```python
from build123d import *

# Parameters (mm, degrees)
BOSS_EXTRUDE1_DEPTH = 550
SKETCH2_W           = 99.516911358
SKETCH2_H           = 250
CUT_EXTRUDE1_DEPTH  = 596.064959308
SKETCH4_R           = 5
CUT_EXTRUDE2_DEPTH  = 20
SKETCH4_3_R         = 5
BOSS_EXTRUDE3_DEPTH = 2.5
BOSS_EXTRUDE4_START = 17.5
SKETCH4_5_R         = 5
BOSS_EXTRUDE4_DEPTH = 2.5
SKETCH4_7_R         = 1.240896304
BOSS_EXTRUDE5_DEPTH = 17.5
BOSS_EXTRUDE6_START = -150
SKETCH5_R           = 5
SKETCH5_R_2         = 1.5
BOSS_EXTRUDE6_DEPTH = 19.5
CUT_EXTRUDE5_START  = -167.5
SKETCH5_4_R         = 5
CUT_EXTRUDE5_DEPTH  = 2.5
CUT_EXTRUDE6_START  = -150
SKETCH5_6_R         = 5
CUT_EXTRUDE6_DEPTH  = 2.5
BOSS_EXTRUDE7_DEPTH = 2


with BuildPart() as part:
    # Sketch1 → Boss-Extrude1 (new body)
    with BuildSketch(Plane.XY):
        Polygon((0, 0), (-63.508529611, 110), (-61.222529611, 110), (0.966177285, 2.286), (200, 2.286), (200, 0), align=None)
    extrude(amount=BOSS_EXTRUDE1_DEPTH)

    # Sketch2 → Cut-Extrude1 (cut, through all)
    with BuildSketch(Plane(origin=(0, 2.286, 0), x_dir=(1, 0, 0), z_dir=(0, 1, 0))):
        with Locations((150.241544321, -275)):
            Rectangle(SKETCH2_W, SKETCH2_H)
    extrude(amount=-CUT_EXTRUDE1_DEPTH, mode=Mode.SUBTRACT)

    # Sketch4 → Cut-Extrude2 (cut)
    with BuildSketch(Plane.XY.offset(150)):
        with Locations((0.483088642, 1.143)):
            Circle(SKETCH4_R)
    cut_extrude2 = extrude(amount=CUT_EXTRUDE2_DEPTH, mode=Mode.SUBTRACT)

    # Sketch4_3 → Boss-Extrude3 (add)
    with BuildSketch(Plane.XY.offset(150)):
        with Locations((0.483088642, 1.143)):
            Circle(SKETCH4_3_R)
    boss_extrude3 = extrude(amount=BOSS_EXTRUDE3_DEPTH)

    # Sketch4_5 → Boss-Extrude4 (add)
    with BuildSketch(Plane.XY.offset(150).offset(BOSS_EXTRUDE4_START)):
        with Locations((0.483088642, 1.143)):
            Circle(SKETCH4_5_R)
    boss_extrude4 = extrude(amount=BOSS_EXTRUDE4_DEPTH)

    # Sketch4_7 → Boss-Extrude5 (add)
    with BuildSketch(Plane.XY.offset(150)):
        with Locations((0.483088642, 1.143)):
            Circle(SKETCH4_7_R)
    boss_extrude5 = extrude(amount=BOSS_EXTRUDE5_DEPTH)

    # Mirror1: Cut-Extrude2, Boss-Extrude3, Boss-Extrude4, Boss-Extrude5 across plane
    add(cut_extrude2.mirror(Plane.XY.offset(275)), mode=Mode.SUBTRACT)
    add(boss_extrude3.mirror(Plane.XY.offset(275)))
    add(boss_extrude4.mirror(Plane.XY.offset(275)))
    add(boss_extrude5.mirror(Plane.XY.offset(275)))

    # Sketch5 → Boss-Extrude6 (add)
    with BuildSketch(Plane.XY.offset(550).offset(BOSS_EXTRUDE6_START)):
        with Locations((-65.55265663, 107.5)):
            Circle(SKETCH5_R)
        with Locations((-65.55265663, 107.5)):
            Circle(SKETCH5_R_2, mode=Mode.SUBTRACT)
    boss_extrude6 = extrude(amount=-BOSS_EXTRUDE6_DEPTH)

    # Sketch5_4 → Cut-Extrude5 (cut)
    with BuildSketch(Plane.XY.offset(550).offset(CUT_EXTRUDE5_START)):
        with Locations((-65.55265663, 107.5)):
            Circle(SKETCH5_4_R)
    cut_extrude5 = extrude(amount=-CUT_EXTRUDE5_DEPTH, mode=Mode.SUBTRACT)

    # Sketch5_6 → Cut-Extrude6 (cut)
    with BuildSketch(Plane.XY.offset(550).offset(CUT_EXTRUDE6_START)):
        with Locations((-65.55265663, 107.5)):
            Circle(SKETCH5_6_R)
    cut_extrude6 = extrude(amount=-CUT_EXTRUDE6_DEPTH, mode=Mode.SUBTRACT)

    # Mirror2: Boss-Extrude6, Cut-Extrude5, Cut-Extrude6 across plane
    add(boss_extrude6.mirror(Plane.XY.offset(275)))
    add(cut_extrude5.mirror(Plane.XY.offset(275)), mode=Mode.SUBTRACT)
    add(cut_extrude6.mirror(Plane.XY.offset(275)), mode=Mode.SUBTRACT)

    # Sketch7 → Boss-Extrude7 (add)
    with BuildSketch(Plane.XY.offset(550)):
        with BuildLine():
            Line((32.714, 2.286), (35, 2.286))
            Line((35, 2.286), (35, 20))
            Line((35, 20), (15, 20))
            Line((15, 20), (19.696699141, 15.303300859))
            ThreePointArc((19.696699141, 15.303300859), (27.870125743, 16.929096494), (32.5, 10))
            ThreePointArc((32.5, 10), (31.929096494, 7.129874257), (30.303300859, 4.696699141))
            Line((30.303300859, 4.696699141), (32.714, 2.286))
        make_face()
        with BuildLine():
            Line((15, 20), (15, 2.286))
            Line((15, 2.286), (32.714, 2.286))
            Line((32.714, 2.286), (30.303300859, 4.696699141))
            ThreePointArc((30.303300859, 4.696699141), (19.696699141, 4.696699141), (19.696699141, 15.303300859))
            Line((19.696699141, 15.303300859), (15, 20))
        make_face()
        Polygon((15, 2.286), (15, 0), (35, 0), (32.714, 2.286), align=None)
        Polygon((32.714, 2.286), (35, 0), (35, 2.286), align=None)
    extrude(amount=BOSS_EXTRUDE7_DEPTH)


solid = part.part
```
Design review of the part built by this model. Coordinates are the model's own, in mm. A direction names the side the tool comes from. Coordinates: 2 decimals unless noted, no trailing zeros. Order: outer loops, then holes, each group sorted by start corner. A loop starts at its lowest first (then second) coordinate and runs counter-clockwise, first axis right, second up.
1) Mouldability with a two-part tool opening along Z and no side actions: class faces 3 (the flat face through (-33, 59, 550)), 4 (the flat face through (20, 17, 550)), 5 (the flat face through (2, 0, 382.5)) as +Z half, -Z half, draft (parallel to the pull), parting line (faces both ways), or undercut.
2) Wall thickness on line 1 along Z through (x, y) = (-45, 81.5); line 2 along Y through (x, z) = (101, 437); line 3 along X through (y, z) = (107.5, 161.25): over which ranges is each line inside the solid? List them lowest first.
3) Take a section at B-B, the plane z = 253.5. Give the boundary of the cut face in (x, y), and give its area (3 significant figures).
4) Take a section at D-D, the plane z = 110. Give the boundary of the cut face in (x, y), and give its area (3 significant figures).
5) Clearance check with flat-ended pins moving along their axes: pin 1 (1 mm diameter, centred on y = 93.5, z = 118, fed in from +X); pin 2 (0.7 mm diameter, centred on y = 1, z = 225.5, fed in from +X); pin 3 (2.5 mm diameter, centred on x = 168.5, y = 0.5, fed in from +Z); pin 4 (3.5 mm diameter, centred on x = -61.5, y = 107, fed in from -Z). State where each tip first meets the part, or that it passes through.
6) Take a section at C-C, the plane x = 169.5. Give the boundary of the cut face in (y, z), and give its area (3 significant figures).
7) For faces 1 (the flat face through (2, 0, 152.5)), 2 (the flat face through (29, 17, 552)), list the 3-axis set-ups (+Z, -Z, +X, -X, +Y, -Y) from which the entire face can be reached by the end or side of a thin tool; tool diameter is ignored.
8) Take a section at A-A, the plane x = 25. Give the boundary of the cut face in (y, z).
Returned:
1. face 3: +Z half
1. face 4: -Z half
1. face 5: undercut
2. line 1: z = 0 to 550
2. line 2: y = 0 to 2.29
2. line 3: x = -70.55 to -67.05, -64.05 to -59.78
3. outline: (-63.51, 110) - (0, 0) - (100.48, 0) - (100.48, 2.29) - (0.97, 2.29) - (-61.22, 110) - close
3. area: 477 mm2
4. outline: (-63.51, 110) - (0, 0) - (200, 0) - (200, 2.29) - (0.97, 2.29) - (-61.22, 110) - close
4. area: 705 mm2
5. pin 1: stops at x = -51.41
5. pin 2: stops at x = 100.48
5. pin 3: stops at z = 550
5. pin 4: stops at z = 0
6. outline: (0, 0) - (2.29, 0) - (2.29, 150) - (0, 150) - close; (0, 400) - (2.29, 400) - (2.29, 550) - (0, 550) - close
6. area: 686 mm2
7. face 1: none
7. face 2: +Z, +X, -X, +Y, -Y
8. outline: (0, 0) - (2.29, 0) - (2.29, 550) - (2.5, 550) - (2.5, 552) - (0, 552) - close; (17.5, 550) - (20, 550) - (20, 552) - (17.5, 552) - close
